Autodesk Inventor part; units mm, degrees
ref_plane "YZ Plane" through (0, 0, 0) normal (1, 0, 0) x (0, 1, 0)
ref_plane "XZ Plane" through (0, 0, 0) normal (0, 1, 0) x (-1, 0, 0)
ref_plane "XY Plane" through (0, 0, 0) normal (0, 0, 1) x (1, 0, 0)
sketch "Sketch1" plane through (0, 0, 0) normal (0, 1, 0) x (-1, 0, 0)
  circle A0 centre (0, 0) radius 7.5
  dimension "d0" = 15
extrude "Extrusion1" add sketch "Sketch1" along normal blind 12.5
sketch "Sketch2" plane through (0, 12.5, 0) normal (0, 1, 0) x (1, 0, 0)
  circle A0 centre (0, 0) radius 7.5
  circle A1 centre (0, 0) radius 9.525
  dimension "d3" = 19.05
extrude "Extrusion2" add sketch "Sketch2" along normal blind 2.5 contours A0 | A1
sketch "Sketch3" plane through (0, 15, 0) normal (0, 1, 0) x (1, 0, 0)
  circle A0 centre (0, 0) radius 9.525
  circle A1 centre (0, 0) radius 3.3
  dimension "d6" = 6.6
extrude "Extrusion3" cut sketch "Sketch3" against normal blind 17.75 contours A1
sketch "Sketch4" plane through (0, 0, 0) normal (0, -1, 0) x (1, 0, 0)
  circle A0 centre (0, 0) radius 3.3
  circle A1 centre (0, 0) radius 7.5
  circle A2 centre (0, 0) radius 5
  dimension "d9" = 10
extrude "Extrusion4" cut sketch "Sketch4" against normal blind 11 contours A2
thread "Thread1"
properties part number "Isolator"
CAD build for the part. Positions are in the model's coordinates, mm. A direction names the side the tool comes from. Give positions to 0.01 mm unless a question says otherwise; leave off trailing zeros. Order: outer loops, then holes, each group sorted by start corner. A loop starts at its lowest first (then second) coordinate and runs counter-clockwise, first axis right, second up. Notation, with made-up numbers: (-28.75, 48) -> (2.25, 48) arc R27 cw to (2.25, 74) -> close; hole circle Ø5 at (64.25, 65.25). An arc over 180 degrees is marked (long way). Return JSON: item names as keys, results as strings.
Q1. Saw through at B-B (x = 0). Write the cut outline in (y, z) (3 decimals).
Working result:
{"outline": "(0, -7.5) -> (12.5, -7.5) -> (12.5, -9.525) -> (15, -9.525) -> (15, -3.3) -> (11, -3.3) -> (11, -5) -> (0, -5) -> close; (0, 5) -> (11, 5) -> (11, 3.3) -> (15, 3.3) -> (15, 9.525) -> (12.5, 9.525) -> (12.5, 7.5) -> (0, 7.5) -> close"}
Q2. Flat gauge pins, fed straight in: pin 1 (2 mm diameter, centred on x = 1, y = 10, fed in from -Z); pin 2 (1 mm diameter, centred on y = 6.5, z = -5, fed in from -X); pin 3 (1.5 mm diameter, centred on y = 1.5, z = -1.5, fed in from -X). Where does each tip first touch, or does it go through?
Working result:
{"pin 1": "z = -7.5", "pin 2": "x = -6", "pin 3": "x = -7.46"}
Q3. Drill centre lines: line 1 (Z direction, x = 0, y = 7.25); line 2 (Z direction, x = 0, y = 14.15) (3 decimals). Where is each one in solid material? Low to high.
Working result:
{"line 1": "-7.5 to -5, 5 to 7.5", "line 2": "-9.525 to -3.3, 3.3 to 9.525"}
Q4. Saw through at D-D (x = 6.5). Write the cut outline in (y, z).
Working result:
{"outline": "(0, -3.74) -> (12.5, -3.74) -> (12.5, -6.96) -> (15, -6.96) -> (15, 6.96) -> (12.5, 6.96) -> (12.5, 3.74) -> (0, 3.74) -> close"}
Q5. Saw through at C-C (y = 13.5). Write the cut outline in (x, z) (3 decimals).
Working result:
{"outline": "circle Ø19.05 at (0, 0); hole circle Ø6.6 at (0, 0)"}
Q6. Which spindle directions (+Z, -Z, +X, -X, +Y, -Y) get a long thin tool onto all of the face, cutting with end or side? Do faces 1 (the face through (-1.08, 5.42, -4.88)), 2 (the face through (-7.559, 13.732, -5.796)). Say none if no direction does.
Working result:
{"face 1": "-Y", "face 2": "+Y, -Y"}
Q7. Saw through at A-A (z = 0). Write the cut outline in (x, y) (3 decimals), then the cut area to 3 significant figures.
Working result:
{"outline": "(-9.525, 12.5) -> (-7.5, 12.5) -> (-7.5, 0) -> (-5, 0) -> (-5, 11) -> (-3.3, 11) -> (-3.3, 15) -> (-9.525, 15) -> close; (3.3, 11) -> (5, 11) -> (5, 0) -> (7.5, 0) -> (7.5, 12.5) -> (9.525, 12.5) -> (9.525, 15) -> (3.3, 15) -> close", "area": "98.7 mm²"}
Q8. Mould opens along X. For faces 3 (the face through (0, 12.5, 8)), 4 (the face through (3.3, 11, 1.2)), 5 (the face through (7.493, 6.162, -0.33)) say: pulls with the +X half, pulls with the -X half, needs draft (parallel to the pull), parting line crosses it, or undercut.
Working result:
{"face 3": "needs draft", "face 4": "undercut", "face 5": "parting line crosses it"}
